Geometry: final body of the model. Coordinates: model frame, mm. A direction names the side the tool comes from. Coordinates: 2 decimals unless noted, no trailing zeros. Order: outer loops, then holes, each group sorted by start corner. A loop starts at its lowest first (then second) coordinate and runs counter-clockwise, first axis right, second up. Notation, with made-up numbers: M 14,-36 L 32,-36 A22 cw 32,-7 Z; hole C 48,83.25 d11. An arc over 180 degrees is marked long. Write item = value, one per line.
from build123d import *

# Parameters (mm, degrees)
SKETCH1_W           = 10
SKETCH1_H           = 10
BOSS_EXTRUDE1_DEPTH = 50
SKETCH2_R           = 3
CUT_EXTRUDE1_DEPTH  = 20
LPATTERN1_COUNT     = 2
LPATTERN1_PITCH     = 30


with BuildPart() as part:
    # Sketch1 → Boss-Extrude1 (new body)
    with BuildSketch(Plane(origin=(0, 0, 0), x_dir=(1, 0, 0), z_dir=(0, 1, 0))):
        Rectangle(SKETCH1_W, SKETCH1_H)
    extrude(amount=BOSS_EXTRUDE1_DEPTH)

    # Sketch2 → Cut-Extrude1 (cut)
    with BuildSketch(Plane.XZ):
        with Locations(Location((0, 0, 0), (0, 0, 270))):
            Circle(SKETCH2_R)
    cut_extrude1 = extrude(amount=-CUT_EXTRUDE1_DEPTH, mode=Mode.SUBTRACT)

    # LPattern1: Cut-Extrude1 ×2
    with Locations(*[(0, i * LPATTERN1_PITCH, 0) for i in range(1, LPATTERN1_COUNT)]):
        add(cut_extrude1, mode=Mode.SUBTRACT)


solid = part.part
1) Mould query, pull axis X, two halves, no side actions, for faces 1 (the face through (0, 30, 0)), 2 (the face through (5, 25, 0)), 3 (the face through (0.9, 39.86, -2.86)), 4 (the face through (0, 25, -5)). Classes: pulls with the +X half, pulls with the -X half, needs draft (parallel to the pull), parting line crosses it, or undercut.
Numbers:
face_1 = undercut
face_2 = pulls with the +X half
face_3 = undercut
face_4 = needs draft
2) Section A-A, the plane z = 0. Return loops of the section in (x, y).
Numbers:
outline = M -5,0 L -3,0 L -3,20 L 3,20 L 3,0 L 5,0 L 5,50 L 3,50 L 3,30 L -3,30 L -3,50 L -5,50 Z
3) Line query: L1, parallel to X at y = 40.75, z = 0; L2, parallel to Y at x = 2.75, z = -0.75; L3, parallel to X at y = 31, z = 2.5. Output: solid intervals per line, ascending.
Numbers:
L1 = -5 to -3, 3 to 5
L2 = 20 to 30
L3 = -5 to -1.66, 1.66 to 5
4) Section B-B, the plane y = 44. Return loops of the section in (x, z).
Numbers:
outline = M -5,-5 L 5,-5 L 5,5 L -5,5 Z; hole C 0,0 d6
5) Section C-C, the plane x = 0. Return loops of the section in (y, z), and give its area (3 significant figures).
Numbers:
outline = M 0,-5 L 50,-5 L 50,-3 L 30,-3 L 30,3 L 50,3 L 50,5 L 0,5 L 0,3 L 20,3 L 20,-3 L 0,-3 Z
area = 260 mm²
6) Pin query (flat end, axial travel): pin 1 (5.5 mm diameter, centred on x = 0, z = 0, fed in from -Y); pin 2 (3 mm diameter, centred on x = 1, z = 0, fed in from +Y). Return the tip coordinate at first contact, or that it passes through.
Numbers:
pin_1 = 20
pin_2 = 30
7) Set-up query: faces 5 (the face through (0, 25, 5)), 6 (the face through (0, 20, 0)). Return all of +Z, -Z, +X, -X, +Y, -Y with unobstructed straight access to the full face (end or side cutting, diameter ignored); none if empty.
Numbers:
face_5 = +Z, +X, -X, +Y, -Y
face_6 = -Y
